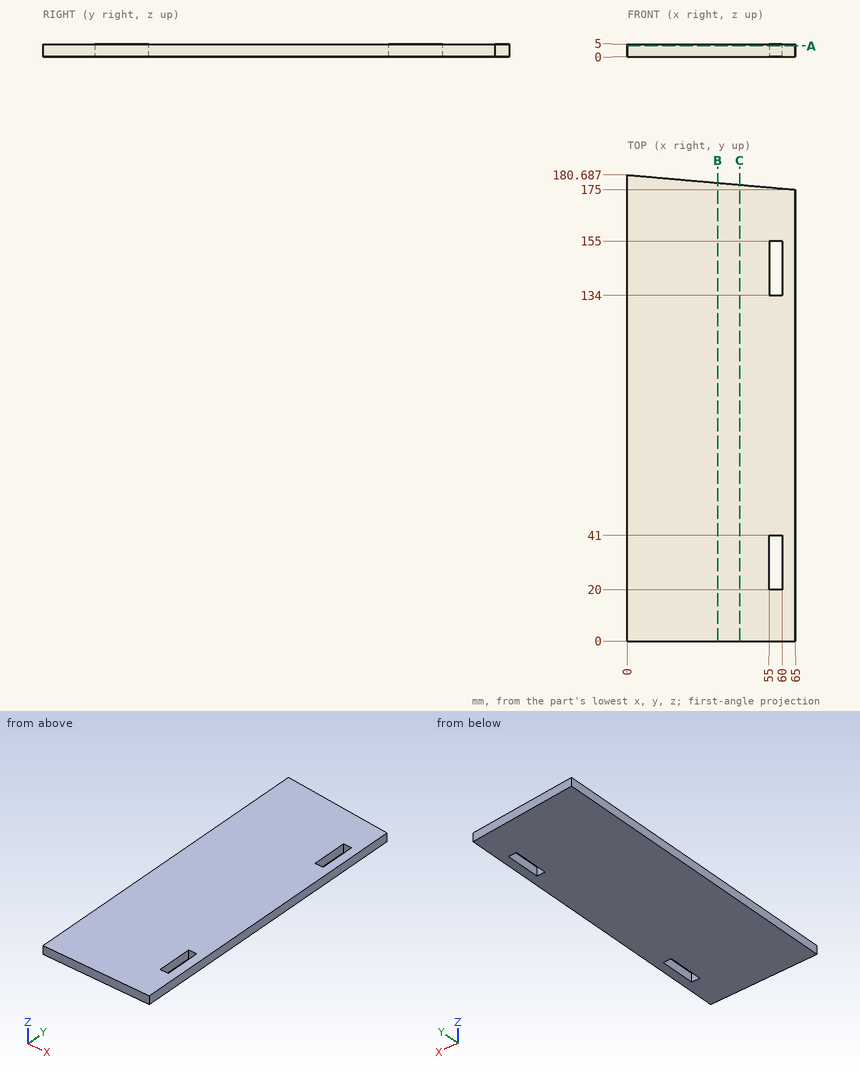
The figure shows three views and two pictorial views of one solid part (mm, origin at its lowest corner). Answer the questions. Round coordinates to 2 decimals unless told otherwise and drop trailing zeros. Write each loop counter-clockwise with the first axis right and the second up, starting at its lowest first coordinate (ties: lowest second). Pieces come first, ordered by that corner, then holes. Notation, with made-up numbers: (58.25, -4.75) - (97.25, -4.75) arc R36 cw to (97.25, 30.25) - close; hole circle Ø6 at (-29, 67.25). An arc over 180 degrees is marked (long way). Use one line per item in the form item = value. Start each with the question number.
Item 1: Find the intervals of material crossed by line 1 (X direction, y = 23, z = 1.2); line 2 (Y direction, x = 57.5, z = 0.65); line 3 (Y direction, x = 22, z = 1.75), in increasing order. Write a range as [from, to].
Item 2: A flat-ended cylindrical pin translates along its axis: pin 1 Ø1.5 at (x, z) = (56.5, 1.5) entering from +Y. Find the tip coordinate at first contact, or state that the pin passes through.
Item 3: A cutting plane is placed at A-A (z = 4.25). Write down the section's boundary in (x, y), plus the area to 4 significant figures.
Item 4: A cutting plane is placed at B-B (x = 35). Write down the section's boundary in (y, z) (1 decimal), plus the area to 3 significant figures.
Item 5: A cutting plane is placed at C-C (x = 43.5). Write down the section's boundary in (y, z).
The answers:
q1.line_1 = [0, 55], [60, 65]
q1.line_2 = [0, 20], [41, 134], [155, 175.66]
q1.line_3 = [0, 178.76]
q2.pin_1 = 175.81
q3.outline = (0, 0) - (65, 0) - (65, 175) - (0, 180.69) - close; hole (55, 20) - (60, 20) - (60, 41) - (55, 41) - close; hole (55, 134) - (60, 134) - (60, 155) - (55, 155) - close
q3.area = 11,350 mm^2
q4.outline = (0, 0) - (177.6, 0) - (177.6, 5) - (0, 5) - close
q4.area = 888 mm^2
q5.outline = (0, 0) - (176.88, 0) - (176.88, 5) - (0, 5) - close
